Can you work these out from the model? Positions are in its coordinate system, mm. Face numbers are marked on the shaded views. A direction names the side the tool comes from. Round coordinates to 2 decimals unless told otherwise and drop trailing zeros. Order: outer loops, then holes, each group sorted by start corner. A loop starts at its lowest first (then second) coordinate and runs counter-clockwise, first axis right, second up.
Q1. If I drill on line 1 (Y direction, x = 36, z = -2.5); line 2 (X direction, y = 16.25, z = -4); line 3 (Y direction, x = -3, z = -1.5), over which ranges is the centre line in solid material (lowest first)?
Q2. If we section it at A-A (z = -2.5): Please give me the cut outline in (x, y), plus the area to 3 significant figures.
Q3. Will these pins go through, and if not, where does the flat tip stop? P1, Ø1.2, axis at x = 29, y = 7, coming from the -Z side; P2, Ø4, axis at x = 14, y = 8.5, coming from the -Z side (3 decimals); P3, Ø4.5, axis at x = 3, y = 19, coming from the -Z side.
Q4. We'd pull the mould along X, two halves only. Please class the marked faces 3, 4, 5 and 6: pulls with the +X half, pulls with the -X half, needs draft (parallel to the pull), parting line crosses it, or undercut.
Q5. If we section it at C-C (x = 21.5): Please give me the cut outline in (y, z) (3 decimals).
Q6. If we section it at B-B (z = 6.25): Please give me the cut outline in (x, y).
Q7. For the marked faces 1 and 2, which set-ups out of +Z, -Z, +X, -X, +Y, -Y let a thin tool reach every point of the face, with its end or its side?
Q8. If we section it at D-D (x = -3): Please give me the cut outline in (y, z).
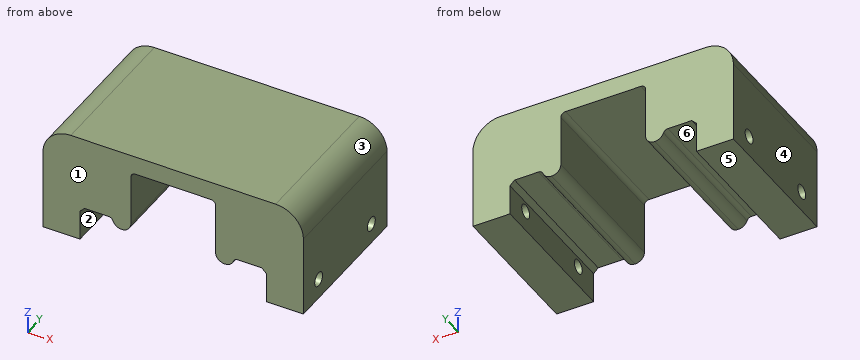
from build123d import *

# Parameters (mm, degrees)
BOSS_EXTRUDE1_DEPTH           = 25.4
CHAMFER1_SIZE                 = 0.79375
SKETCH4_W                     = 1.2
SKETCH4_H                     = 6.35
M2_CLEARANCE_HOLE1_AT_2_COUNT = 2
M2_CLEARANCE_HOLE1_AT_2_PITCH = 16
FILLET1_R                     = 4.7625
FILLET5_R                     = 1.5875
FILLET6_R                     = 1.5875
FILLET7_R                     = 0.79375
SKETCH6_W                     = 1.2
SKETCH6_H                     = 6.35
M2_CLEARANCE_HOLE2_AT_2_COUNT = 2
M2_CLEARANCE_HOLE2_AT_2_PITCH = 16


with BuildPart() as part:
    # Sketch1 → Boss-Extrude1 (new body)
    with BuildSketch(Plane(origin=(0, 0, 0), x_dir=(1, 0, 0), z_dir=(0, 1, 0))):
        with BuildLine():
            Line((0, 0), (0, 5.9944))
            Line((0, 5.9944), (-6.35, 5.9944))
            Line((-6.35, 5.9944), (-6.35, -12.7))
            Line((-6.35, -12.7), (38.354, -12.7))
            Line((38.354, -12.7), (38.354, 5.9944))
            Line((38.354, 5.9944), (32.004, 5.9944))
            Line((32.004, 5.9944), (32.004, 0))
            Line((32.004, 0), (26.44775, 0))
            Line((26.44775, 0), (26.44775, 1.5875))
            Line((26.44775, 1.5875), (23.27275, 1.5875))
            Line((23.27275, 1.5875), (23.27275, -8.73125))
            ThreePointArc((23.27275, -8.73125), (23.040266008, -9.292516008), (22.479, -9.525))
            Line((22.479, -9.525), (9.525, -9.525))
            ThreePointArc((9.525, -9.525), (8.963733992, -9.292516008), (8.73125, -8.73125))
            Line((8.73125, -8.73125), (8.73125, 1.5875))
            Line((8.73125, 1.5875), (5.55625, 1.5875))
            Line((5.55625, 1.5875), (5.55625, 0))
            Line((5.55625, 0), (0, 0))
        make_face()
    extrude(amount=BOSS_EXTRUDE1_DEPTH)

    # Chamfer1
    chamfer1_edges = [part.edges().sort_by_distance(p)[0] for p in [
        (0, 12.7, 0),
        (32.004, 12.7, 0),
    ]]
    chamfer(chamfer1_edges, length=CHAMFER1_SIZE)

    # Sketch4 → M2 Clearance Hole1 (revolve, cut)
    with BuildSketch(Plane(origin=(0, 20.6390625, -2.5), x_dir=(0, 0, -1), z_dir=(0, 1, 0))):
        with Locations((0.6, 3.175)):
            Rectangle(SKETCH4_W, SKETCH4_H)
    m2_clearance_hole1 = revolve(axis=Axis((6.35, 20.6390625, -2.5), (-1, 0, 0)), mode=Mode.SUBTRACT)

    # M2 Clearance Hole1 at 2: M2 Clearance Hole1 ×2
    with Locations(*[(0, -i * M2_CLEARANCE_HOLE1_AT_2_PITCH, 0) for i in range(1, M2_CLEARANCE_HOLE1_AT_2_COUNT)]):
        add(m2_clearance_hole1, mode=Mode.SUBTRACT)

    # Fillet1
    fillet1_edges = [part.edges().sort_by_distance(p)[0] for p in [
        (-6.35, 12.7, 12.7),
        (38.354, 12.7, 12.7),
    ]]
    fillet(fillet1_edges, radius=FILLET1_R)

    # Fillet5
    fillet5_edges = [part.edges().sort_by_distance(p)[0] for p in [
        (5.55625, 12.7, -1.5875),
        (8.73125, 12.7, -1.5875),
    ]]
    fillet(fillet5_edges, radius=FILLET5_R - 0.0001)  # a hair under: the kernel refuses the full size

    # Fillet6
    fillet6_edges = [part.edges().sort_by_distance(p)[0] for p in [
        (23.27275, 12.7, -1.5875),
        (26.44775, 12.7, -1.5875),
    ]]
    fillet(fillet6_edges, radius=FILLET6_R - 0.0001)  # a hair under: the kernel refuses the full size

    # Fillet7
    fillet7_edges = [part.edges().sort_by_distance(p)[0] for p in [
        (5.55625, 12.7, 0),
        (26.44775, 12.7, 0),
    ]]
    fillet(fillet7_edges, radius=FILLET7_R)

    # Sketch6 → M2 Clearance Hole2 (revolve, cut)
    with BuildSketch(Plane(origin=(32.004, 4.6390625, -2.5), x_dir=(0, 0, 1), z_dir=(0, 1, 0))):
        with Locations((0.6, 3.175)):
            Rectangle(SKETCH6_W, SKETCH6_H)
    m2_clearance_hole2 = revolve(axis=Axis((25.654, 4.6390625, -2.5), (1, 0, 0)), mode=Mode.SUBTRACT)

    # M2 Clearance Hole2 at 2: M2 Clearance Hole2 ×2
    with Locations(*[(0, i * M2_CLEARANCE_HOLE2_AT_2_PITCH, 0) for i in range(1, M2_CLEARANCE_HOLE2_AT_2_COUNT)]):
        add(m2_clearance_hole2, mode=Mode.SUBTRACT)


solid = part.part
Solution:
1. line 1: y = 0 to 3.44, 5.84 to 19.44, 21.84 to 25.4
1. line 2: x = -6.35 to 0, 32 to 38.35
1. line 3: y = 0 to 3.98, 5.3 to 19.98, 21.3 to 25.4
2. outline: (-6.35, 0) - (0, 0) - (0, 3.44) - (-6.35, 3.44) - close; (-6.35, 5.84) - (0, 5.84) - (0, 19.44) - (-6.35, 19.44) - close; (-6.35, 21.84) - (0, 21.84) - (0, 25.4) - (-6.35, 25.4) - close; (32, 0) - (38.35, 0) - (38.35, 3.44) - (32, 3.44) - close; (32, 5.84) - (38.35, 5.84) - (38.35, 19.44) - (32, 19.44) - close; (32, 21.84) - (38.35, 21.84) - (38.35, 25.4) - (32, 25.4) - close
2. area: 262 mm2
3. P1: stops at z = 0
3. P2: stops at z = 9.525
3. P3: stops at z = -0.08
4. face 3: pulls with the +X half
4. face 4: pulls with the -X half
4. face 5: needs draft
4. face 6: undercut
5. outline: (0, 9.525) - (25.4, 9.525) - (25.4, 12.7) - (0, 12.7) - close
6. outline: (-6.35, 0) - (8.73, 0) - (8.73, 25.4) - (-6.35, 25.4) - close; (23.27, 0) - (38.35, 0) - (38.35, 25.4) - (23.27, 25.4) - close
7. face 1: +Z, -Z, +X, -X, -Y
7. face 2: -Z, +Y, -Y
8. outline: (0, -5.99) - (25.4, -5.99) - (25.4, 12.49) - (0, 12.49) - close; hole circle Ø2.4 at (4.64, -2.5); hole circle Ø2.4 at (20.64, -2.5)
